from build123d import *

# Parameters (mm, degrees)
EXTRUDE_1_DEPTH = 1.6
EXTRUDE_2_DEPTH = 0.75


with BuildPart() as part:
    # ｽｹｯﾁ1 → ﾎﾞｽ - 押し出し1 (new body)
    with BuildSketch(Plane(origin=(0, 0, 0), x_dir=(1, 0, 0), z_dir=(0, 1, 0))):
        Polygon((0, 255), (42.438235274, 257.290455594), (5, 0), (-5, 0), (-42.438235274, 257.290455594), align=None)
    extrude(amount=EXTRUDE_1_DEPTH)

    # ｽｹｯﾁ2 → ﾎﾞｽ - 押し出し2 (add, symmetric)
    with BuildSketch(Plane(origin=(0, 0, 0), x_dir=(0, 0, -1), z_dir=(1, 0, 0))):
        Polygon((0, 0), (0, -5), (247.53787589, -40), (257.290455594, 0), align=None)
    extrude(amount=EXTRUDE_2_DEPTH, both=True)


solid = part.part
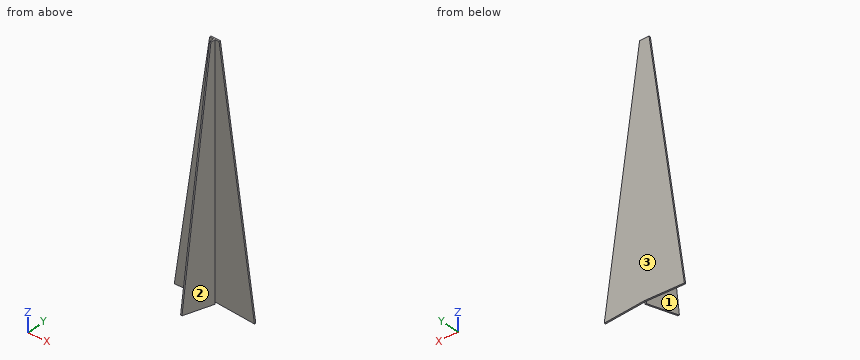
Could you check a few things on this model? Use its own coordinates, in mm. Face numbers are marked on the shaded views. A direction names the side the tool comes from. Coordinates: 2 decimals unless noted, no trailing zeros. Order: outer loops, then holes, each group sorted by start corner. A loop starts at its lowest first (then second) coordinate and runs counter-clockwise, first axis right, second up. Notation, with made-up numbers: (89.25, -18.5) -> (99.25, -18.5) arc R18 ccw to (99.25, -9.5) -> close; hole circle Ø9 at (36, 70.5). An arc over 180 degrees is marked (long way). One line per item, written item: value. Start each with the question number.
1) Imagine slicing it at C-C on x = -18.5. List the corners of the cut face in (y, z) for me.
2) Which directions (+Z, -Z, +X, -X, +Y, -Y) give clear straight access to the entire face, cutting with the end or side of a thin tool? Please do the marked faces 1, 2 and 3.
3) Imagine slicing it at A-A on z = -28.5. List the corners of the cut face in (x, y) for me.
4) Imagine slicing it at B-B on y = -28.5. List the corners of the cut face in (x, z) for me, plus the area to 3 significant figures.
5) I'm going to push flat-ended pins straight in: pin 1 (1.5 mm diameter, centred on x = 18, z = -222, fed in from -Y); pin 2 (1 mm diameter, centred on y = -21.5, z = -109.5, fed in from -X); pin 3 (12 mm diameter, centred on y = -18.5, z = -146.5, fed in from -X); pin 4 (20 mm diameter, centred on y = -18, z = -142, fed in from +X). Where does each tip first touch, or does it pass through?
6) If I drill on L1, parallel to X at y = -15, z = -90; L2, parallel to Y at x = 6, z = -124, over which ranges is the centre line in solid material (lowest first)? Write a range as [from, to].
7) Imagine slicing it at D-D on z = -187. List the corners of the cut face in (x, y) for me.
Answer list:
1. outline: (0, -256) -> (1.6, -256) -> (1.6, -92.78) -> (0, -92.78) -> close
2. face 1: +Z, -Z, -X, -Y
2. face 2: +Z, -Z, +X, -Y
2. face 3: +Z, -Z, +X, -X, +Y
3. outline: (-9.15, 0) -> (-0.75, 0) -> (-0.75, -9.03) -> (0.75, -9.03) -> (0.75, 0) -> (9.15, 0) -> (9.15, 1.6) -> (-9.15, 1.6) -> close
4. outline: (-0.75, -250.34) -> (0.75, -250.34) -> (0.75, -166.2) -> (-0.75, -166.2) -> close
4. area: 126 mm2
5. pin 1: stops at y = 0
5. pin 2: passes through
5. pin 3: stops at x = -0.75
5. pin 4: stops at x = 0.75
6. L1: x = [-0.75, 0.75]
6. L2: y = [0, 1.6]
7. outline: (-32.21, 0) -> (-0.75, 0) -> (-0.75, -31.44) -> (0.75, -31.44) -> (0.75, 0) -> (32.21, 0) -> (32.21, 1.6) -> (-32.21, 1.6) -> close
